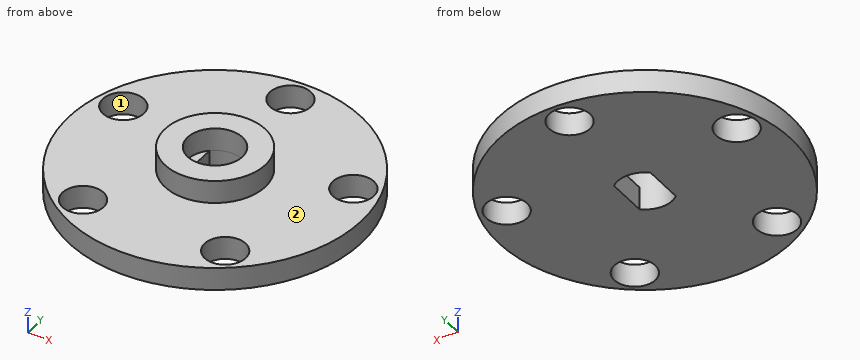
from build123d import *

# Parameters (mm, degrees)
CUT_EXTRUDE1_DEPTH = 5
SKETCH3_R          = 32
SKETCH3_R_2        = 11
CUT_EXTRUDE2_DEPTH = 5
SKETCH4_R          = 4.5
CUT_EXTRUDE3_DEPTH = 5


with BuildPart() as part:
    # Sketch1 → Revolve1 (revolve)
    with BuildSketch(Plane(origin=(0, 0, 0), x_dir=(1, 0, 0), z_dir=(0, 1, 0))):
        Polygon((4, 10), (32, 10), (32, 0), (6, 0), (6, 5), (4, 5), align=None)
    revolve(axis=Axis((0, 0, 0), (0, 0, -1)))

    # Sketch2 → Cut-Extrude1 (cut)
    with BuildSketch(Plane(origin=(0, 0, -10), x_dir=(-1, 0, 0), z_dir=(0, 0, -1))):
        with BuildLine():
            Line((-4, 4.472135955), (-4, -4.472135955))
            ThreePointArc((-4, -4.472135955), (0, -6), (4, -4.472135955))
            Line((4, -4.472135955), (4, 4.472135955))
            ThreePointArc((4, 4.472135955), (0, 6), (-4, 4.472135955))
        make_face()
    extrude(amount=-CUT_EXTRUDE1_DEPTH, mode=Mode.SUBTRACT)

    # Sketch3 → Cut-Extrude2 (cut)
    with BuildSketch(Plane.XY):
        Circle(SKETCH3_R)
        Circle(SKETCH3_R_2, mode=Mode.SUBTRACT)
    extrude(amount=-CUT_EXTRUDE2_DEPTH, mode=Mode.SUBTRACT)

    # Sketch4 → Cut-Extrude3 (cut)
    with BuildSketch(Plane.XY.offset(-5)):
        with Locations((0, 26.5)):
            Circle(SKETCH4_R)
        with Locations((25.202997682, 8.188950351)):
            Circle(SKETCH4_R)
        with Locations((15.576309186, -21.438950351)):
            Circle(SKETCH4_R)
        with Locations((-15.576309186, -21.438950351)):
            Circle(SKETCH4_R)
        with Locations((-25.202997682, 8.188950351)):
            Circle(SKETCH4_R)
    extrude(amount=-CUT_EXTRUDE3_DEPTH, mode=Mode.SUBTRACT)


solid = part.part
Geometry: final body of the model. Coordinates: model frame, mm. Face numbers are marked on the shaded views. A direction names the side the tool comes from. Give positions to 0.01 mm unless a question says otherwise; leave off trailing zeros. Write each loop counter-clockwise with the first axis right and the second up, starting at its lowest first coordinate (ties: lowest second). Pieces come first, ordered by that corner, then holes. Notation, with made-up numbers: M -27,-30.5 L 10,-30.5 A38 cw 10,7.5 Z; hole C 22,-22.75 d8. An arc over 180 degrees is marked long. Answer in a Markdown table with one row per item. Add a question column.
(1) Section A-A on x = 0. Return loops of the section in (y, z), and give its area (3 significant figures).
(2) Reachability of the marked faces 1 and 2 from +Z, -Z, +X, -X, +Y, -Y: full face, straight path, thin tool, end or side. Return the list, or none.
(3) Section D-D on z = -7.75. Return loops of the section in (x, y).
(4) First-contact query: pin 1 (6 mm diameter, centred on x = -23.5, y = 23.5, fed in from +Z); pin 2 (5.5 mm diameter, centred on x = 0, y = 26.5, fed in from -Z); pin 3 (2 mm diameter, centred on x = 20, z = -6.5, fed in from +Y); pin 4 (6 mm diameter, centred on y = -14, z = -5, fed in from -X). Flat tips, straight axial feed; report the tip coordinate or a pass-through.
(5) Section C-C on x = 26.5. Return loops of the section in (y, z), and give its area (3 significant figures).
(6) Ray query, line 1 (X direction, y = 10, z = -9); line 2 (Y direction, x = 1.5, z = -7); line 3 (Z direction, x = -16.5, y = 22). Return the intervals inside material, ascending.
(7) Section B-B on y = 0. Return loops of the section in (x, z).
Result set:
| question | item | result |
|---|---|---|
| 1 | outline | M -32,-10 L -6,-10 L -6,0 L -11,0 L -11,-5 L -32,-5 Z; M 6,-10 L 22,-10 L 22,-5 L 11,-5 L 11,0 L 6,0 Z; M 31,-10 L 32,-10 L 32,-5 L 31,-5 Z |
| 1 | area | 265 mm^2 |
| 2 | face 1 | +Z, -Z |
| 2 | face 2 | +Z |
| 3 | outline | C 0,0 d64; hole C -25.2,8.19 d9; hole C -15.58,-21.44 d9; hole C 0,26.5 d9; hole M -4,-4.47 A6 ccw 4,-4.47 L 4,4.47 A6 ccw -4,4.47 Z; hole C 15.58,-21.44 d9; hole C 25.2,8.19 d9 |
| 4 | pin 1 | stops at z = -5 |
| 4 | pin 2 | passes through |
| 4 | pin 3 | stops at y = 25.75 |
| 4 | pin 4 | stops at x = -30.05 |
| 5 | outline | M -17.94,-10 L 3.88,-10 L 3.88,-5 L -17.94,-5 Z; M 12.5,-10 L 17.94,-10 L 17.94,-5 L 12.5,-5 Z |
| 5 | area | 136 mm^2 |
| 6 | line 1 | x = -30.4 to -29.32, -21.08 to 21.08, 29.32 to 30.4 |
| 6 | line 2 | y = -31.96 to -5.81, 5.81 to 22.26, 30.74 to 31.96 |
| 6 | line 3 | z = -10 to -5 |
| 7 | outline | M -32,-10 L -4,-10 L -4,-5 L -6,-5 L -6,0 L -11,0 L -11,-5 L -32,-5 Z; M 4,-10 L 32,-10 L 32,-5 L 11,-5 L 11,0 L 6,0 L 6,-5 L 4,-5 Z |
